Could you check a few things on this model? Use its own coordinates, in mm. Face numbers are marked on the shaded views. A direction names the side the tool comes from. Coordinates: 2 decimals unless noted, no trailing zeros. Loops run counter-clockwise (first coordinate to the right, second up) from the corner with the lowest first, then second, coordinate; pieces in that order, holes last.
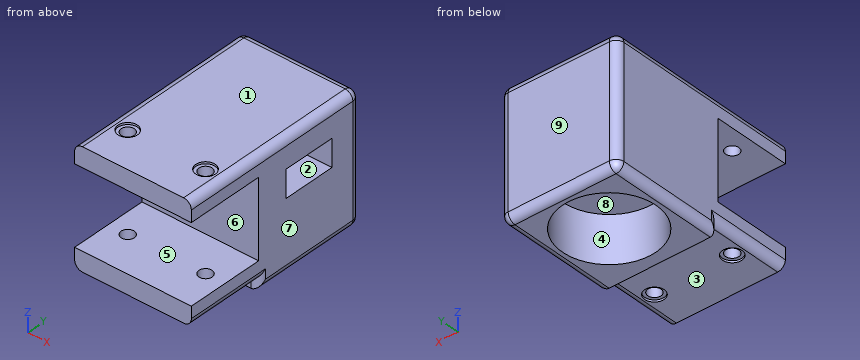
from build123d import *

# Parameters (mm, degrees)
SKETCH1_W               = 30
SKETCH1_H               = 50
BOSS_EXTRUDE1_DEPTH     = 15
SKETCH6_W               = 30
SKETCH6_H               = 30
BOSS_EXTRUDE2_DEPTH     = 2.5
SKETCH2_W               = 30
SKETCH2_H               = 20
CUT_EXTRUDE1_DEPTH      = 20
SKETCH3_R               = 1.7
CUT_EXTRUDE2_DEPTH      = 28.5
CUT_EXTRUDE2_DEPTH_BACK = 6
SKETCH5_W               = 7
SKETCH5_H               = 13.6
CUT_EXTRUDE5_DEPTH      = 22.8
CUT_EXTRUDE8_START      = -4.5
SKETCH3_4_R             = 2.5
CUT_EXTRUDE8_DEPTH      = 0.5
MIRROR4_START           = -4.5
MIRROR4_COPY_1_SKETCH_R = 2.5
MIRROR4_COPY_1_DEPTH    = 0.5
FILLET1_R               = 2
SKETCH7_R               = 4.5
SKETCH7_R_2             = 12
CUT_EXTRUDE9_DEPTH      = 12
CUT_EXTRUDE10_REACH     = 34.5
SKETCH7_4_R             = 4.5


with BuildPart() as part:
    # Sketch1 → Boss-Extrude1 (new body, symmetric)
    with BuildSketch(Plane.XY):
        Rectangle(SKETCH1_W, SKETCH1_H)
    extrude(amount=BOSS_EXTRUDE1_DEPTH, both=True)

    # Sketch6 → Boss-Extrude2 (add)
    with BuildSketch(Plane(origin=(0, 0, -15), x_dir=(-1, 0, 0), z_dir=(0, 0, -1))):
        with Locations((0, 10)):
            Rectangle(SKETCH6_W, SKETCH6_H)
    extrude(amount=BOSS_EXTRUDE2_DEPTH)

    # Sketch2 → Cut-Extrude1 (cut)
    with BuildSketch(Plane.XZ.offset(25)):
        Rectangle(SKETCH2_W, SKETCH2_H)
    extrude(amount=-CUT_EXTRUDE1_DEPTH, mode=Mode.SUBTRACT)

    # Sketch3 → Cut-Extrude2 (cut, two sides)
    with BuildSketch(Plane(origin=(0, 0, 10), x_dir=(-1, 0, 0), z_dir=(0, 0, -1))) as cut_extrude2_sk:
        with Locations((-10, -15)):
            Circle(SKETCH3_R)
        with Locations((10, -15)):
            Circle(SKETCH3_R)
    extrude(amount=CUT_EXTRUDE2_DEPTH, mode=Mode.SUBTRACT)
    extrude(cut_extrude2_sk.sketch, amount=-CUT_EXTRUDE2_DEPTH_BACK, mode=Mode.SUBTRACT)

    # Sketch5 → Cut-Extrude5 (cut)
    with BuildSketch(Plane(origin=(15, 0, 0), x_dir=(0, 0, -1), z_dir=(1, 0, 0))):
        with Locations((-4, 10)):
            Rectangle(SKETCH5_W, SKETCH5_H)
    extrude(amount=-CUT_EXTRUDE5_DEPTH, mode=Mode.SUBTRACT)

    # Sketch3<4> → Cut-Extrude8 (cut)
    with BuildSketch(Plane(origin=(0, 0, 10), x_dir=(-1, 0, 0), z_dir=(0, 0, -1)).offset(CUT_EXTRUDE8_START)):
        with Locations((-10, -15)):
            Circle(SKETCH3_4_R)
    cut_extrude8 = extrude(amount=-CUT_EXTRUDE8_DEPTH, mode=Mode.SUBTRACT)

    # Mirror3: Cut-Extrude8 across plane
    add(cut_extrude8.mirror(Plane(origin=(0, 0, 0), x_dir=(0, 0, 1), z_dir=(1, 0, 0))), mode=Mode.SUBTRACT)

    # Mirror4: Cut-Extrude8 across plane
    add(cut_extrude8.mirror(Plane.XY), mode=Mode.SUBTRACT)

    # Mirror4 copy 1 sketch → Mirror4 copy 1 (cut)
    with BuildSketch(Plane.XY.offset(-10).offset(MIRROR4_START)):
        with Locations((-10, -15)):
            Circle(MIRROR4_COPY_1_SKETCH_R)
    extrude(amount=-MIRROR4_COPY_1_DEPTH, mode=Mode.SUBTRACT)

    # Fillet1
    fillet1_edges = [part.edges().sort_by_distance(p)[0] for p in [
        (15, 0, 15),
        (0, 25, 15),
        (-15, -15, -15),
        (-15, -5, -16.25),
        (15, -5, -16.25),
        (-15, 10, -17.5),
        (0, 25, -17.5),
        (15, 10, -17.5),
        (-15, 0, 15),
        (15, -15, -15),
        (-15, 25, -1.25),
        (15, 25, -1.25),
    ]]
    fillet(fillet1_edges, radius=FILLET1_R)

    # Sketch7 → Cut-Extrude9 (cut)
    with BuildSketch(Plane(origin=(0, 0, -17.5), x_dir=(-1, 0, 0), z_dir=(0, 0, -1))):
        with Locations((0, 10)):
            Circle(SKETCH7_R)
        with Locations((0, 10)):
            Circle(SKETCH7_R_2)
        with Locations((0, 10)):
            Circle(SKETCH7_R, mode=Mode.SUBTRACT)
    extrude(amount=-CUT_EXTRUDE9_DEPTH, mode=Mode.SUBTRACT)

    # Sketch7<4> → Cut-Extrude10 (cut, up to next)
    with BuildSketch(Plane(origin=(0, 0, -17.5), x_dir=(-1, 0, 0), z_dir=(0, 0, -1)), mode=Mode.PRIVATE) as cut_extrude10_sk1:
        with Locations((0, 10)):
            Circle(SKETCH7_4_R)
    cut_extrude10_tool1 = extrude(cut_extrude10_sk1.sketch, amount=-CUT_EXTRUDE10_REACH, mode=Mode.PRIVATE) & part.part
    add(cut_extrude10_tool1.solids().sort_by_distance((0, 10, -17.5))[0], mode=Mode.SUBTRACT)


solid = part.part
1) Imagine slicing it at C-C on z = 2. List the corners of the cut face in (x, y) for me, plus the area to 3 significant figures.
2) We'd pull the mould along Y, two halves only. Please class the marked faces 6, 7, 8 and 9: released by +Y, released by -Y, zero draft, split by the parting line, or undercut.
3) Imagine slicing it at A-A on y = 10. List the corners of the cut face in (x, z) for me, plus the area to 3 significant figures.
4) For the marked faces 1, 2, 3, 4 and 5, which set-ups out of +Z, -Z, +X, -X, +Y, -Y let a thin tool reach every point of the face, with its end or its side?
5) Imagine slicing it at B-B on x = -10. State how many separate pieces and enclosed holes the cut face has, plus the area to 3 significant figures.
6) If I drill on L1, parallel to Y at x = 8.5, z = 2.5; L2, parallel to Z at x = 0.5, y = -8; L3, parallel to Z at x = 6.25, y = 10.5, over which ranges is the centre line in solid material (lowest first)?
7) Will these pins go through, and if not, where does the flat tip stop? pin 1 (2.5 mm diameter, centred on x = -10, y = -15.5, fed in from +Z); pin 2 (6 mm diameter, centred on x = -7, y = 11.5, fed in from -Z); pin 3 (1.5 mm diameter, centred on x = 10, y = -15.5, fed in from -Z); pin 4 (12 mm diameter, centred on x = 11, z = 1, fed in from -Y).
8) Imagine slicing it at D-D on x = -5.25. List the corners of the cut face in (y, z) for me, plus the area to 3 significant figures.
Solved:
1. outline: (-15, -5) - (15, -5) - (15, 3.2) - (-7.8, 3.2) - (-7.8, 16.8) - (15, 16.8) - (15, 23) arc R2 ccw to (13, 25) - (-13, 25) arc R2 ccw to (-15, 23) - close
1. area: 588 mm2
2. face 6: released by -Y
2. face 7: zero draft
2. face 8: undercut
2. face 9: released by +Y
3. outline: (-15, -15.5) arc R2 ccw to (-13, -17.5) - (-12, -17.5) - (-12, -5.5) - (-4.5, -5.5) - (-4.5, 0.5) - (-7.8, 0.5) - (-7.8, 7.5) - (15, 7.5) - (15, 13) arc R2 ccw to (13, 15) - (-13, 15) arc R2 ccw to (-15, 13) - close; (4.5, -5.5) - (12, -5.5) - (12, -17.5) - (13, -17.5) arc R2 ccw to (15, -15.5) - (15, 0.5) - (4.5, 0.5) - close
3. area: 470 mm2
4. face 1: +Z, +X, -X, +Y, -Y
4. face 2: +X
4. face 3: -Z, +X, -X, -Y
4. face 4: -Z
4. face 5: +X, -X, -Y
5. separate pieces: 3
5. enclosed holes: 0
5. area: 978 mm2
6. L1: y = -5 to 3.2, 16.8 to 25
6. L2: z = -15 to -10, 10 to 15
6. L3: z = -5.5 to 0.5, 7.5 to 15
7. pin 1: stops at z = 14.5
7. pin 2: stops at z = -5.5
7. pin 3: passes through
7. pin 4: stops at y = -5
8. outline: (-25, -15) - (-5, -15) - (-5, -17.5) - (-0.79, -17.5) - (-0.79, -5.5) - (20.79, -5.5) - (20.79, -17.5) - (23, -17.5) arc R2 ccw to (25, -15.5) - (25, 13) arc R2 ccw to (23, 15) - (-25, 15) - (-25, 10) - (-5, 10) - (-5, -10) - (-25, -10) - close; hole (3.2, 0.5) - (16.8, 0.5) - (16.8, 7.5) - (3.2, 7.5) - close
8. area: 819 mm2
